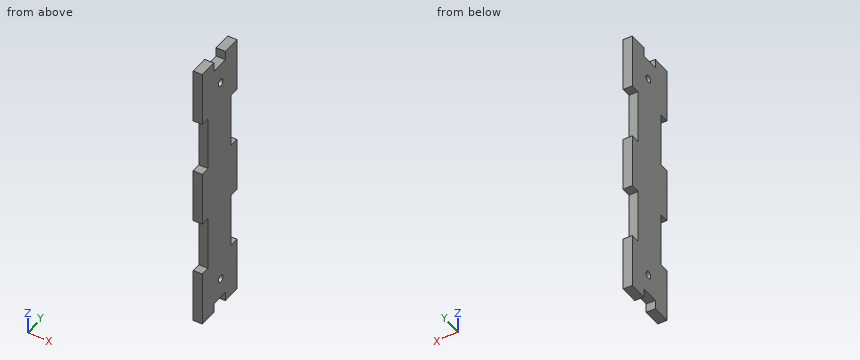
from build123d import *

# Parameters (mm, degrees)
CROQUIS1_R              = 2
SALIENTE_EXTRUIR1_DEPTH = 5


with BuildPart() as part:
    # Croquis1 → Saliente-Extruir1 (new body)
    with BuildSketch(Plane(origin=(0, 0, 0), x_dir=(0, 0, -1), z_dir=(1, 0, 0))):
        Polygon((0, 20), (5, 20), (5, 10), (0, 10), (0, 0), (30, 0), (30, 5), (60, 5), (60, 0), (90, 0), (90, 5), (120, 5), (120, 0), (150, 0), (150, 10), (145, 10), (145, 20), (150, 20), (150, 30), (120, 30), (120, 25), (90, 25), (90, 30), (60, 30), (60, 25), (30, 25), (30, 30), (0, 30), align=None)
        with Locations((16, 16)):
            Circle(CROQUIS1_R, mode=Mode.SUBTRACT)
        with Locations(Location((134, 16, 0), (0, 0, 180))):
            Circle(CROQUIS1_R, mode=Mode.SUBTRACT)
    extrude(amount=SALIENTE_EXTRUIR1_DEPTH)


solid = part.part
Geometry check sheet. Reference: the model listing, model coordinates, mm. Round coordinates to 2 decimals unless told otherwise and drop trailing zeros. Order: outer loops, then holes, each group sorted by start corner. A loop starts at its lowest first (then second) coordinate and runs counter-clockwise, first axis right, second up. Notation, with made-up numbers: M 62.25,11 L 111.25,11 A24 cw 111.25,46 Z; hole C 66,40.25 d6. An arc over 180 degrees is marked long. Answer in a Markdown table with one row per item.
(1) Sectioned sample at B-B, the plane z = -16. Record the cut outline in (x, y), and give its area (3 significant figures).
Responses:
| item | result |
|---|---|
| outline | M 0,0 L 5,0 L 5,14 L 0,14 Z; M 0,18 L 5,18 L 5,30 L 0,30 Z |
| area | 130 mm² |
(2) Sectioned sample at A-A, the plane y = 16. Record the cut outline in (x, z), and give its area (3 significant figures).
Responses:
| item | result |
|---|---|
| outline | M 0,-145 L 5,-145 L 5,-136 L 0,-136 Z; M 0,-132 L 5,-132 L 5,-18 L 0,-18 Z; M 0,-14 L 5,-14 L 5,-5 L 0,-5 Z |
| area | 660 mm² |
(3) Sectioned sample at D-D, the plane y = 28. Record the cut outline in (x, z), and give its area (3 significant figures).
Responses:
| item | result |
|---|---|
| outline | M 0,-150 L 5,-150 L 5,-120 L 0,-120 Z; M 0,-90 L 5,-90 L 5,-60 L 0,-60 Z; M 0,-30 L 5,-30 L 5,0 L 0,0 Z |
| area | 450 mm² |
(4) Sectioned sample at C-C, the plane x = 3.8. State how many separate pieces and enclosed holes the cut face has, and give its area (3 significant figures).
Responses:
| item | result |
|---|---|
| separate pieces | 1 |
| enclosed holes | 2 |
| area | 3,770 mm² |
(5) Go/stop test with flat-tipped pins: P1, Ø2.5, axis at x = 2, y = 17, coming from the -Z side; P2, Ø1, axis at x = 3, z = -92.5, coming from the -Y side; P3, Ø2.5, axis at x = 3, z = -103, coming from the +Y side. Record where each tip stops, or that it passes through.
Responses:
| item | result |
|---|---|
| P1 | stops at z = -145 |
| P2 | stops at y = 5 |
| P3 | stops at y = 25 |
(6) Scan lines: probe 1 along Z at (x, y) = (2.4, 3); probe 2 along Y at (x, z) = (2.8, -134); probe 3 along Z at (x, y) = (3.7, 14.5). Record each from-to range of solid material in increasing order. Write a range as from..to.
Responses:
| item | result |
|---|---|
| probe 1 | z = -150..-120, -90..-60, -30..0 |
| probe 2 | y = 0..14, 18..30 |
| probe 3 | z = -145..-135.32, -132.68..-17.32, -14.68..-5 |
